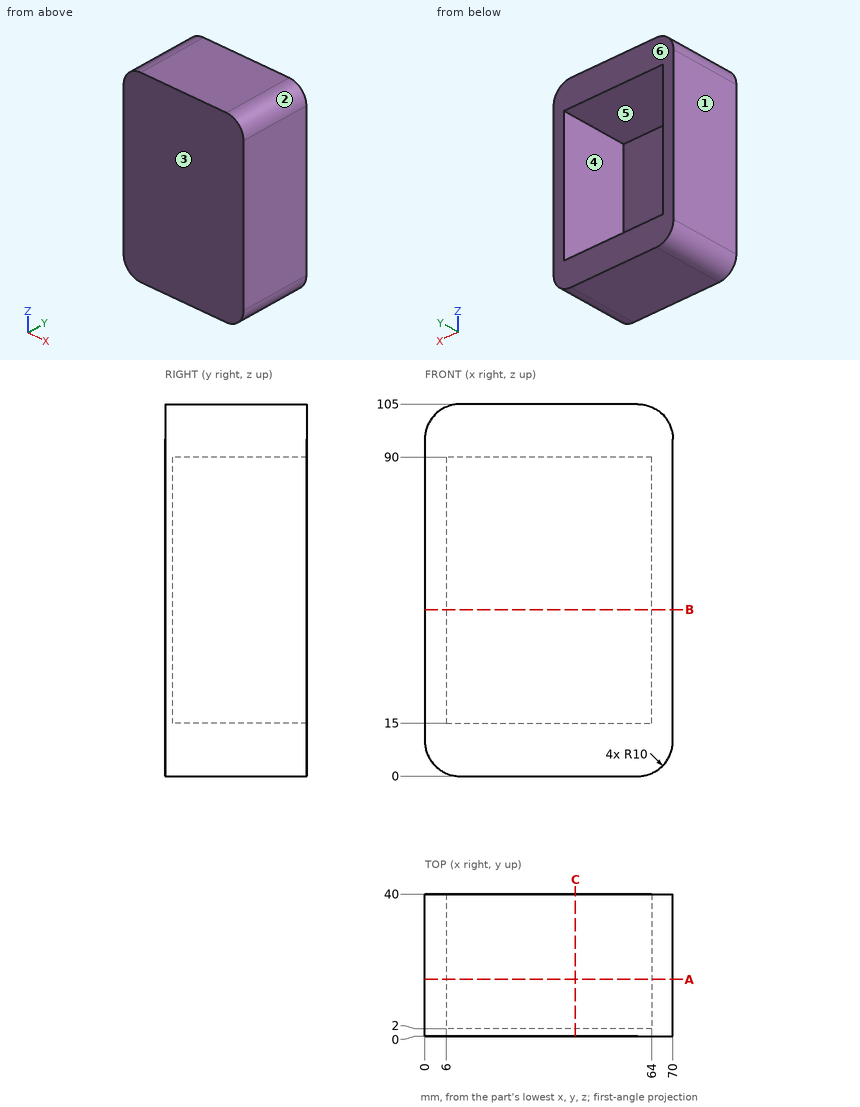
Job drawing, mm, ordinate dimensions from the low corner. One solid piece. A direction names the side the tool comes from. Give positions to 0.01 mm unless a question says otherwise; leave off trailing zeros. Loops run counter-clockwise (first coordinate to the right, second up) from the corner with the lowest first, then second, coordinate; pieces in that order, holes last. Notation, with made-up numbers: (16, -26.5) - (20, -26.5) arc R19 cw to (20, 0.5) - close; hole circle Ø5 at (48, -6). An arc over 180 degrees is marked (long way). Use one line per item in the form item = value.
(1) Cut at A-A (y = 16). Give the cut face in (x, z), then the cut area to 3 significant figures.
Determined:
outline = (0, 10) arc R10 ccw to (10, 0) - (60, 0) arc R10 ccw to (70, 10) - (70, 95) arc R10 ccw to (60, 105) - (10, 105) arc R10 ccw to (0, 95) - close; hole (6, 15) - (64, 15) - (64, 90) - (6, 90) - close
area = 2,910 mm^2
(2) Cut at C-C (x = 42.5). Give the cut face in (y, z).
Determined:
outline = (0, 0) - (40, 0) - (40, 15) - (2, 15) - (2, 90) - (40, 90) - (40, 105) - (0, 105) - close
(3) Pull direction X, two halves, no side cores. Call the marked faces 1, 2, 3 and 4: pulls with the +X half, pulls with the -X half, needs draft (parallel to the pull), parting line crosses it, or undercut.
Determined:
face_1 = pulls with the -X half
face_2 = pulls with the +X half
face_3 = needs draft
face_4 = undercut
(4) Drop a flat-ended pin along its axis: P1, Ø8, axis at x = 17, z = 75, coming from the +Y side. Give the stop position or say it passes through.
Determined:
P1 = 2
(5) Drill centre lines: L1, parallel to X at y = 37, z = 55; L2, parallel to Z at x = 54.5, y = 4.5; L3, parallel to Y at x = 36.5, z = 64.5. Where is each one in solid material? Low to high.
Determined:
L1 = 0 to 6, 64 to 70
L2 = 0 to 15, 90 to 105
L3 = 0 to 2
(6) Cut at B-B (z = 47). Give the cut face in (x, y), then the cut area to 3 significant figures.
Determined:
outline = (0, 0) - (70, 0) - (70, 40) - (64, 40) - (64, 2) - (6, 2) - (6, 40) - (0, 40) - close
area = 596 mm^2
(7) 3-axis set-ups, long thin cutter, end or side, ignore diameter. For the marked faces 5 and 6: which of +Z, -Z, +X, -X, +Y, -Y reach the whole face in a straight line?
Determined:
face_5 = +Y
face_6 = +Z, -Z, +X, -X, +Y
